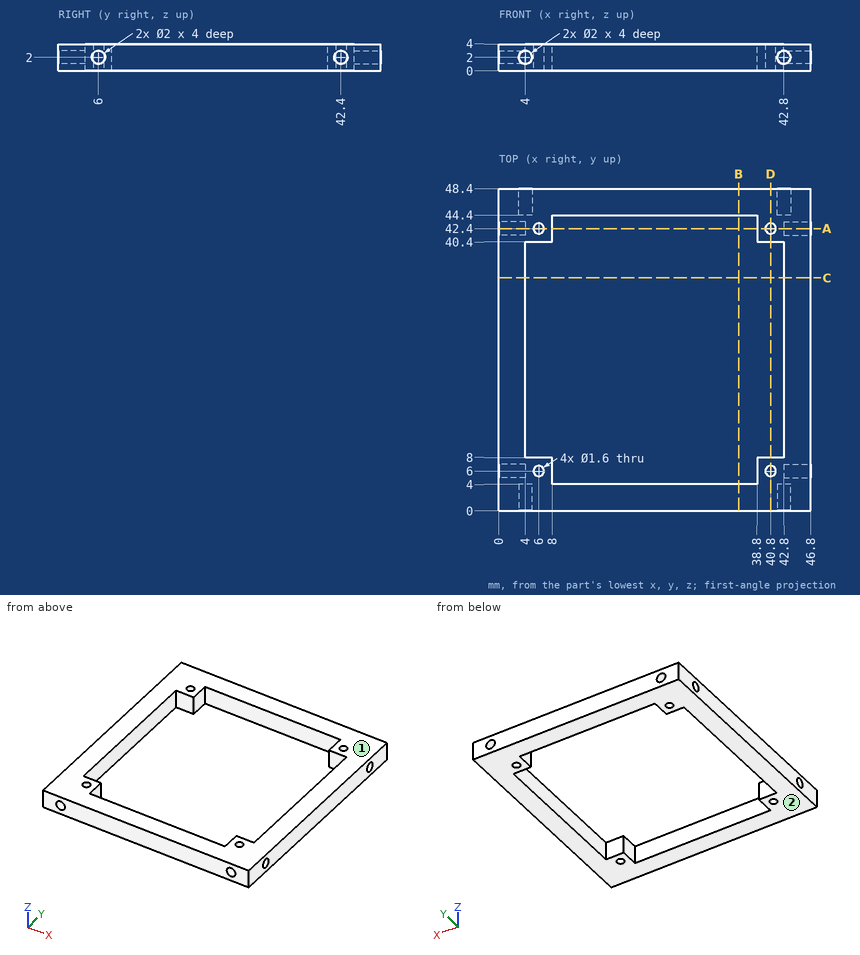
Geometry check sheet. Reference: drawing and pictorial views, mm from the part's lowest x, y, z. Give positions to 0.01 mm unless a question says otherwise; leave off trailing zeros. Order: outer loops, then holes, each group sorted by start corner. A loop starts at its lowest first (then second) coordinate and runs counter-clockwise, first axis right, second up. Notation, with made-up numbers: (-36.75, 70) - (20.25, 70) arc R8 ccw to (20.25, 85) - close; hole circle Ø5 at (62, -33.75). An arc over 180 degrees is marked (long way). Use one line per item in the form item = value.
1) Material ranges on probe 1 along Y at (x, z) = (6, 0.2); probe 2 along Y at (x, z) = (2.5, 2); probe 3 along X at (y, z) = (42.4, 1.9), recorded low to high. Write a range as from..to.
Working result:
probe_1 = 0..5.2, 6.8..8, 40.4..41.6, 43.2..48.4
probe_2 = 0..5, 7..41.4, 43.4..48.4
probe_3 = 4..5.2, 6.8..8, 38.8..40, 41.6..42.8
2) Sectioned sample at A-A (y = 42.4). Record the boundary of the cut face in (x, z).
Working result:
outline = (0, 0) - (5.2, 0) - (5.2, 4) - (0, 4) - (0, 3) - (4, 3) - (4, 1) - (0, 1) - close; (6.8, 0) - (8, 0) - (8, 4) - (6.8, 4) - close; (38.8, 0) - (40, 0) - (40, 4) - (38.8, 4) - close; (41.6, 0) - (46.8, 0) - (46.8, 1) - (42.8, 1) - (42.8, 3) - (46.8, 3) - (46.8, 4) - (41.6, 4) - close
3) Draft check along Z on the marked faces 1 and 2. Enter one of: released by +Z, released by -Z, zero draft, split by the parting line, or undercut.
Working result:
face_1 = released by +Z
face_2 = released by -Z
4) Sectioned sample at B-B (x = 36). Record the boundary of the cut face in (y, z).
Working result:
outline = (0, 0) - (4, 0) - (4, 4) - (0, 4) - close; (44.4, 0) - (48.4, 0) - (48.4, 4) - (44.4, 4) - close
5) Sectioned sample at C-C (y = 35). Record the boundary of the cut face in (x, z).
Working result:
outline = (0, 0) - (4, 0) - (4, 4) - (0, 4) - close; (42.8, 0) - (46.8, 0) - (46.8, 4) - (42.8, 4) - close
6) Sectioned sample at D-D (x = 40.8). Record the boundary of the cut face in (y, z).
Working result:
outline = (0, 0) - (5.2, 0) - (5.2, 4) - (0, 4) - close; (6.8, 0) - (8, 0) - (8, 4) - (6.8, 4) - close; (40.4, 0) - (41.6, 0) - (41.6, 4) - (40.4, 4) - close; (43.2, 0) - (48.4, 0) - (48.4, 4) - (43.2, 4) - close
7) Depth check by flat-ended pin: pin 1 Ø1.6 at (x, z) = (42.8, 2) entering from +Y; pin 2 Ø1.2 at (y, z) = (6, 2) entering from -X; pin 3 Ø1.6 at (y, z) = (42.4, 2) entering from +X. Enter the tip coordinate at first touch or a pass-through.
Working result:
pin_1 = 44.4
pin_2 = 4
pin_3 = 42.8
